Check sheet for the modelled part. Datum: model origin and axes. Units: mm. A direction names the side the tool comes from. Give positions to 0.01 mm unless a question says otherwise; leave off trailing zeros. Order: outer loops, then holes, each group sorted by start corner. A loop starts at its lowest first (then second) coordinate and runs counter-clockwise, first axis right, second up.
from build123d import *

# Parameters (mm, degrees)
F0_R      = 3.275
F1_DEPTH  = 17.5
F3_DEPTH  = 14.526
F5_DEPTH  = 11.1862926682
F7_DEPTH  = 35.001
F8_R      = 0.5
F9_W      = 1.5
F9_H      = 5
F12_DEPTH = 5
F13_SIZE  = 1
F14_R     = 1
F15_R     = 3.275
F16_DEPTH = 1.2


# Not quite as in the source:
# - a pattern or mirror of a feature is missing from the dataset's text; its kind, count and spacing are read off the source's solid
# - a feature names something its author has since deleted; it is built from what else it names


with BuildPart() as f1:
    # F0 (on Front) → F1 (new body, symmetric)
    with BuildSketch(Plane.XZ):
        with BuildLine():
            Line((-6.25, 8.275), (-6.25, 0))
            Line((-6.25, 0), (-2, 0))
            Line((-2, 0), (0, 2))
            Line((0, 2), (2, 0))
            Line((2, 0), (6.25, 0))
            Line((6.25, 0), (6.25, 8.275))
            ThreePointArc((6.25, 8.275), (0, 14.525), (-6.25, 8.275))
        make_face()
        with Locations((0, 8.275)):
            Circle(F0_R, mode=Mode.SUBTRACT)
    extrude(amount=F1_DEPTH, both=True)

    # F2 (on face) → F3 (cut, through all)
    with BuildSketch(Plane(origin=(0, 0, 0), x_dir=(1, 0, 0), z_dir=(0, 0, -1))):
        Polygon((-1.5, -2.5), (-6.25, 2.25), (-6.25, -12.5), (-1.5, -7.75), align=None)
    extrude(amount=-F3_DEPTH, mode=Mode.SUBTRACT)

    # F4 (on face) → F5 (join, through all)
    with BuildSketch(Plane(origin=(0, 0, 0), x_dir=(1, 0, 0), z_dir=(0, 0, -1))):
        Polygon((-4.65, 0.65), (-6.25, 2.25), (-6.25, -11.75), (-2, -7.5), (-4.65, -4.85), align=None)
    extrude(amount=-F5_DEPTH)

    # F6 (on face) → F7 (cut, through all)
    with BuildSketch(Plane.XZ.offset(17.5)):
        with BuildLine():
            Line((-6.25, 11.1862926682), (-6.25, 8.275))
            ThreePointArc((-6.25, 8.275), (-6.0674696664, 9.774437177), (-5.5305402087, 11.1862926682))
            Line((-5.5305402087, 11.1862926682), (-6.25, 11.1862926682))
        make_face()
    extrude(amount=-F7_DEPTH, mode=Mode.SUBTRACT)

    # F8
    f8_edges = [f1.edges().sort_by_distance(p)[0] for p in [
        (-2, 7.5, 5.593146),
    ]]
    fillet(f8_edges, radius=F8_R)

    # F9 (on face) → F10 (revolve, cut)
    with BuildSketch(Plane(origin=(0, 0, 0), x_dir=(1, 0, 0), z_dir=(0, 0, -1))):
        with Locations((-3.75, -13.8)):
            Rectangle(F9_W, F9_H)
    f10 = revolve(axis=Axis((0, 0.2600380681, 0), (0, -1, 0)), mode=Mode.SUBTRACT)

    # F10_copies: F10 across plane
    add(f10.mirror(Plane(origin=(0, 0, 0), x_dir=(0, 0, -1), z_dir=(0, -1, 0))), mode=Mode.SUBTRACT)

    # F11 (on face) → F12 (cut, through all)
    with BuildSketch(Plane(origin=(0, 11.3, 0), x_dir=(-1, 0, 0), z_dir=(0, 1, 0))):
        with BuildLine():
            ThreePointArc((-4.5, 0), (-3.1819805153, 3.1819805153), (0, 4.5))
            Line((0, 4.5), (-3, 4.5))
            Line((-3, 4.5), (-3, 5.2))
            Line((-3, 5.2), (-4.3, 6.5))
            Line((-4.3, 6.5), (-6.25, 6.5))
            Line((-6.25, 6.5), (-6.25, 4.5))
            Line((-6.25, 4.5), (-6.25, 0))
            Line((-6.25, 0), (-4.5, 0))
        make_face()
    f12 = extrude(amount=F12_DEPTH, mode=Mode.SUBTRACT)

    # F12_copies: F12 across plane
    add(f12.mirror(Plane(origin=(0, 0, 0), x_dir=(0, 0, -1), z_dir=(0, -1, 0))), mode=Mode.SUBTRACT)

    # F13
    f13_edges = [f1.edges().sort_by_distance(p)[0] for p in [
        (-6.25, 15, 0),
        (-6.25, -2.875, 0),
        (6.25, 0, 0),
        (6.25, -16.9, 0),
        (6.25, 16.9, 0),
    ]]
    chamfer(f13_edges, length=F13_SIZE)

    # F14
    f14_edges = [f1.edges().sort_by_distance(p)[0] for p in [
        (-1, 17.5, 1),
        (1, 17.5, 1),
        (-1, -17.5, 1),
        (1, -17.5, 1),
        (-6.25, 17.5, 4.6375),
        (0, -17.5, 14.525),
        (0, 17.5, 14.525),
        (6.25, 17.5, 4.6375),
        (-6.25, -17.5, 4.6375),
        (6.25, -17.5, 4.6375),
    ]]
    fillet(f14_edges, radius=F14_R)

    # F15 (on face) → F16 (join)
    with BuildSketch(Plane(origin=(0, 17.5, 0), x_dir=(-1, 0, 0), z_dir=(0, 1, 0))):
        with Locations((0, 8.275)):
            Circle(F15_R)
    extrude(amount=-F16_DEPTH)


solid = f1.part
1) Depth check by flat-ended pin: pin 1 Ø1.5 at (x, y) = (1.5, -15) entering from -Z; pin 2 Ø1.7 at (x, y) = (-4, 6) entering from +Z; pin 3 Ø0.6 at (y, z) = (-14.5, 5) entering from +X; pin 4 Ø1.6 at (y, z) = (5.5, 13) entering from -X. Enter the tip coordinate at first touch or a pass-through.
Recorded:
pin 1: stops at z = 0
pin 2: stops at z = 11.19
pin 3: stops at x = 3.1
pin 4: stops at x = -1.5
2) Section check B-B, the plane y = 13. Record the cut outline in (x, z) (3 decimals).
Recorded:
outline: (-6.25, 1) - (-5.25, 0) - (-4.5, 0) arc R4.5 cw to (0, 4.5) - (3, 4.5) - (3, 5.2) - (4.3, 6.5) - (6.25, 6.5) - (6.25, 8.275) arc R6.25 ccw to (-6.25, 8.275) - close; (-3, 0) - (-2, 0) - (0, 2) - (2, 0) - (3, 0) arc R3 ccw to start; hole circle Ø6.55 at (0, 8.275)
3) Section check C-C, the plane x = 1.25. State how many separate pieces and enclosed holes the cut face has, then the cut area to 3 significant figures.
Recorded:
separate pieces: 1
enclosed holes: 2
area: 254 mm2
4) Set-up check for faces 4 (the face through (-3.147, -13.765, 3.217)), 5 (the face through (-1.284, -17.325, 1.332)), 6 (the face through (-1.5, 5, 13)): record each of +Z, -Z, +X, -X, +Y, -Y from which the full face is reachable in a straight line by a thin tool's end or side.
Recorded:
face 4: none
face 5: -Z, -Y
face 6: +Z, -Z, -X
5) Material ranges on L1, parallel to Y at x = 0.75, z = 3.75; L2, parallel to Y at x = -4, z = 8.25; L3, parallel to Y at x = -5.25, z = 0.5, recorded low to high.
Recorded:
L1: y = -17.5 to -16.3, -11.3 to 11.3, 16.3 to 17.5
L2: y = -17.5 to 0, 5.5 to 9.5, 10.25 to 17.5
L3: y = -17.5 to 10.75, 11.5 to 17.5
6) Section check A-A, the plane y = 6. Record the cut outline in (x, z) (3 decimals), then the cut area to 3 significant figures.
Recorded:
outline: (-6.25, 1) - (-5.25, 0) - (-3.5, 0) - (-3.5, 11.186) - (-5.531, 11.186) arc R6.25 ccw to (-6.25, 8.275) - close; (-1.5, 0.5) - (0, 2) - (2, 0) - (5.25, 0) - (6.25, 1) - (6.25, 8.275) arc R6.25 ccw to (-1.5, 14.342) - (-1.5, 11.186) arc R3.275 cw (long way) to (-1.5, 5.364) - close
area: 103 mm2
7) Draft check along Y on faces 1 (the face through (0, 17.5, 7)), 2 (the face through (-3.5, 6, 5.5)), 3 (the face through (-6.25, -3, 5)). Enter one of: +Y half, -Y half, draft (parallel to the pull), parting line (faces both ways), or undercut.
Recorded:
face 1: +Y half
face 2: undercut
face 3: draft
